Work out the finished part from the listing and answer in its coordinate system (mm). Face numbers are marked on the shaded views. Coordinates: 2 decimals unless noted, no trailing zeros. Order: outer loops, then holes, each group sorted by start corner. A loop starts at its lowest first (then second) coordinate and runs counter-clockwise, first axis right, second up. Notation, with made-up numbers: (-15.5, -30) - (-1.5, -30) arc R7 ccw to (-1.5, -19) - close; hole circle Ø11 at (-35.75, -12). An arc over 180 degrees is marked (long way). Answer as a JSON object with one key per item and string values. Group by question number.
1) Section B-B (z = 26) is taken. Give the vertices of the cut face in (x, y), plus the area to 3 significant figures.
2) The mould has two halves that part along X. Classify the marked faces 1, 2 and 3: released by +X, released by -X, zero draft, split by the parting line, or undercut.
3) Section A-A (x = 195.5) is taken. Give the vertices of the cut face in (y, z).
4) Find the intervals of material crossed by line 1 along Z through (x, y) = (134.5, 57); line 2 along Y through (x, z) = (48, 14); line 3 along X through (y, z) = (53, 105), in increasing order.
5) Each of these flat-tipped pins is pushed along its axis until it touches: P1, Ø2, axis at x = 161, z = 85.5, coming from the -Y side; P2, Ø1.5, axis at y = 59.5, z = 85, coming from the -X side; P3, Ø5, axis at y = 54, z = 81, coming from the -X side. Where does it stop, or does it pass through?
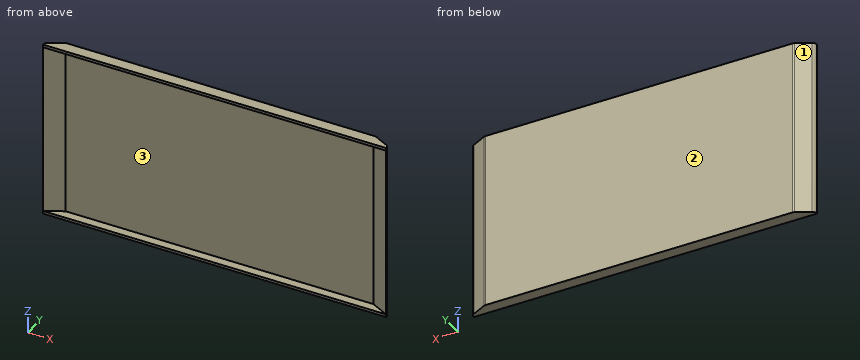
Autodesk Inventor part; units mm, degrees
ref_plane "YZ Plane" through (0, 0, 0) normal (1, 0, 0) x (0, 1, 0)
ref_plane "XZ Plane" through (0, 0, 0) normal (0, 1, 0) x (-1, 0, 0)
ref_plane "XY Plane" through (0, 0, 0) normal (0, 0, 1) x (1, 0, 0)
sketch "Sketch1" plane through (0, 0, 0) normal (0, 0, 1) x (1, 0, 0)
  line L0 (328.3961, 60) -> (-3.3961, 60)
  line L1 (-3.3961, 60) -> (-22.5738, 50.2284)
  line L2 (347.5738, 50.2284) -> (328.3961, 60)
  line L3 (-22.5738, 53.5954) -> (-4.1163, 63)
  line L4 (-4.1163, 63) -> (329.1163, 63)
  line L5 (329.1163, 63) -> (347.5738, 53.5954)
  line L6 (-22.5738, 50.2284) -> (-22.5738, 53.5954)
  line L7 (347.5738, 50.2284) -> (347.5738, 53.5954)
  point P0 (0, 0)
  dimension "d0" = 3
extrude "Extrusion1" add sketch "Sketch1" along normal blind 186.8
sketch "Sketch2" plane through (0, 0, 186.8) normal (0, 0, 1) x (1, 0, 0)
  line L0 (-22.5738, 53.5954) -> (-22.5738, 50.2284)
  line L1 (328.3961, 60) -> (347.5738, 50.2284)
  line L2 (-22.5738, 50.2284) -> (347.5738, 50.2284)
  line L3 (329.1163, 63) -> (-4.1163, 63)
  line L4 (-4.1163, 63) -> (-22.5738, 53.5954)
  line L5 (347.5738, 53.5954) -> (329.1163, 63)
  line L6 (347.5738, 50.2284) -> (347.5738, 53.5954)
  point P0 (0, 0)
extrude "Extrusion2" add sketch "Sketch2" along normal blind 3
sketch "Sketch3" plane through (0, 0, 0) normal (0, 0, -1) x (-1, 0, 0)
  line L0 (-328.3961, 60) -> (-347.5738, 50.2284)
  line L1 (22.5738, 50.2284) -> (-347.5738, 50.2284)
  line L2 (22.5738, 50.2284) -> (3.3961, 60)
  line L3 (3.3961, 60) -> (-328.3961, 60)
  line L4 (-347.5738, 53.5954) -> (-329.1163, 63)
  line L5 (-347.5738, 50.2284) -> (-347.5738, 53.5954)
  line L6 (-347.5738, 53.5954) -> (-329.1163, 63)
  line L7 (-347.5738, 50.2284) -> (-347.5738, 53.5954)
  line L8 (-328.3961, 60) -> (-347.5738, 50.2284)
  line L9 (3.3961, 60) -> (-328.3961, 60)
  line L10 (22.5738, 50.2284) -> (3.3961, 60)
  line L11 (22.5738, 53.5954) -> (22.5738, 50.2284)
  line L12 (4.1163, 63) -> (22.5738, 53.5954)
  line L13 (-329.1163, 63) -> (4.1163, 63)
  point P0 (0, 0)
extrude "Extrusion3" add sketch "Sketch3" along normal blind 3
fillet "Fillet1" radius 5 4 edges at (329.1163, 63, 93.4) (347.5738, 53.5954, 93.4) (-4.1163, 63, 93.4) (-22.5738, 53.5954, 93.4)
properties part number "pokrywa_czołg"
Report:
{
 "1": {"outline": "(-22.57, 50.23) - (-3.4, 60) - (328.4, 60) - (347.57, 50.23) - (347.57, 50.53) arc R5 ccw to (344.84, 54.99) - (330.19, 62.46) arc R5 ccw to (327.92, 63) - (-2.92, 63) arc R5 ccw to (-5.19, 62.46) - (-19.84, 54.99) arc R5 ccw to (-22.57, 50.53) - close", "area": "1,120 mm²"},
 "2": {"face 1": "released by -X", "face 2": "zero draft", "face 3": "undercut"},
 "3": {"outline": "(50.23, -3) - (63, -3) - (63, 189.8) - (50.23, 189.8) - (50.23, 186.8) - (60, 186.8) - (60, 0) - (50.23, 0) - close"},
 "4": {"line 1": "z = -3 to 0, 186.8 to 189.8", "line 2": "y = 60 to 63", "line 3": "x = -21.92 to -17.13, 342.13 to 346.92"},
 "5": {"P1": "stops at y = 60", "P2": "stops at x = -12.46", "P3": "stops at x = -22.48"}
}
